Design review of the part built by this model. Coordinates are the model's own, in mm. Round coordinates to 2 decimals unless told otherwise and drop trailing zeros. Order: outer loops, then holes, each group sorted by start corner. A loop starts at its lowest first (then second) coordinate and runs counter-clockwise, first axis right, second up.
from build123d import *

# Parameters (mm, degrees)
F0_R     = 2.297315
F1_DEPTH = 76.2
F2_W     = 0.757628
F2_H     = 0.697389
F2_W_2   = 0.738942
F2_H_2   = 0.819422
F3_DEPTH = 2.54


with BuildPart() as f1:
    # F0 (on Top) → F1 (new body)
    with BuildSketch(Plane.XY):
        Circle(F0_R)
    extrude(amount=F1_DEPTH)

    # F2 (on Front) → F3 (join)
    with BuildSketch(Plane.XZ):
        with Locations((0, 73.495656)):
            Rectangle(F2_W, F2_H)
        with Locations((0, 3.56264)):
            Rectangle(F2_W_2, F2_H_2)
    extrude(amount=F3_DEPTH)


solid = f1.part
1) Clearance check with flat-ended pins moving along their axes: P1, Ø2, axis at x = 1, z = 43.5, coming from the +Y side; P2, Ø1, axis at x = -1.5, z = 54.5, coming from the +Y side. State where each tip first meets the part, or that it passes through.
Results:
P1: stops at y = 2.3
P2: stops at y = 2.07
2) Take a section at C-C on x = -1.3. Give the boundary of the cut face in (y, z).
Results:
outline: (-1.89, 0) - (1.89, 0) - (1.89, 76.2) - (-1.89, 76.2) - close
3) Take a section at B-B on y = -1.65. Give the boundary of the cut face in (x, z), plus the area to 3 significant figures.
Results:
outline: (-1.6, 0) - (1.6, 0) - (1.6, 76.2) - (-1.6, 76.2) - close
area: 244 mm2
4) Take a section at A-A on z = 28.5. Give the boundary of the cut face in (x, y).
Results:
outline: circle Ø4.59 at (0, 0)
5) To check wall thickness, follow line 1 along Y through (x, z) = (1.4, 45); line 2 along Y through (x, z) = (0.4, 67). State the ranges of each line that lie inside material, in increasing order.
Results:
line 1: y = -1.82 to 1.82
line 2: y = -2.26 to 2.26
